Could you check a few things on this drawing? It's one solid part, dimensions in mm from its lowest x, y, z. A direction names the side the tool comes from. Give positions to 0.01 mm unless a question says otherwise; leave off trailing zeros. Order: outer loops, then holes, each group sorted by start corner. A loop starts at its lowest first (then second) coordinate and runs counter-clockwise, first axis right, second up. Notation, with made-up numbers: (-18.5, 29.25) - (39.5, 29.25) arc R37 ccw to (39.5, 66.25) - close; hole circle Ø10 at (89.5, 19.25). An arc over 180 degrees is marked (long way). Return JSON: item names as keys, results as strings.
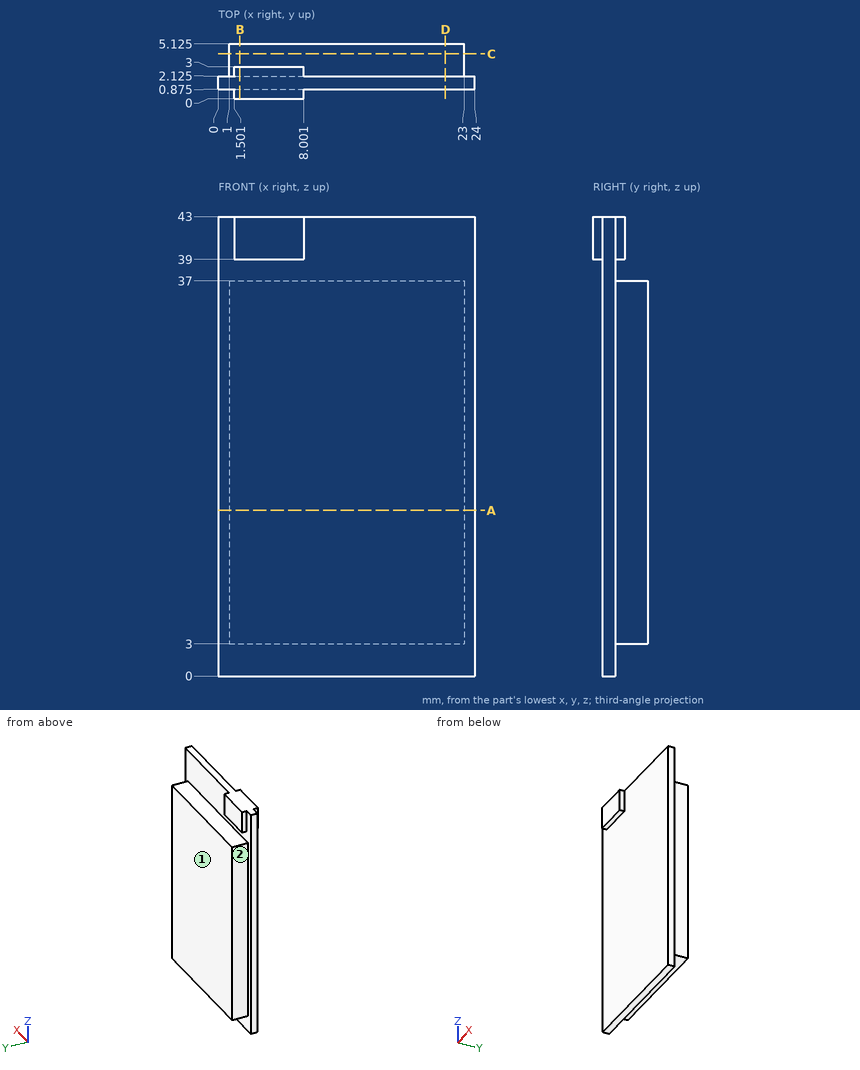
1. Suppose I cut it at A-A (z = 15.5). List the corners of the cut face in (x, y) for me (3 decimals).
Checks:
{"outline": "(0, 0.875) - (24, 0.875) - (24, 2.125) - (23, 2.125) - (23, 5.125) - (1, 5.125) - (1, 2.125) - (0, 2.125) - close"}
2. Suppose I cut it at B-B (x = 2). List the corners of the cut face in (y, z) for me (3 decimals).
Checks:
{"outline": "(0, 39) - (0.875, 39) - (0.875, 0) - (2.125, 0) - (2.125, 3) - (5.125, 3) - (5.125, 37) - (2.125, 37) - (2.125, 39) - (3, 39) - (3, 43) - (0, 43) - close"}
3. If I drill on L1, parallel to Y at x = 10, z = 4.5 (3 decimals); L2, parallel to X at y = 4.85, z = 24.5; L3, parallel to Y at x = 19.5, z = 37.5 (3 decimals), over which ranges is the centre line in solid material (lowest first)? Write a range as [from, to].
Checks:
{"L1": "[0.875, 5.125]", "L2": "[1, 23]", "L3": "[0.875, 2.125]"}
4. Suppose I cut it at D-D (x = 21.25). List the corners of the cut face in (y, z) for me (3 decimals), plus the area to 3 significant figures.
Checks:
{"outline": "(0.875, 0) - (2.125, 0) - (2.125, 3) - (5.125, 3) - (5.125, 37) - (2.125, 37) - (2.125, 43) - (0.875, 43) - close", "area": "156 mm^2"}
5. On a 3-axis mill with a long thin cutter (end or side, diameter ignored), from which of +Z, -Z, +X, -X, +Y, -Y can I reach the whole of each face in a straight line? I mean the marked faces 1 and 2. Say none if no direction works.
Checks:
{"face 1": "+Z, -Z, +X, -X, +Y", "face 2": "+Z, -Z, -X, +Y"}
6. Suppose I cut it at C-C (y = 4.2). List the corners of the cut face in (x, z) for me.
Checks:
{"outline": "(1, 3) - (23, 3) - (23, 37) - (1, 37) - close"}
7. For pin 1 Ø4.5 at (x, z) = (6.5, 40.5) entering from +Y; pin 2 Ø0.9 at (y, z) = (3.5, 26) entering from +X; pin 3 Ø2 at (x, y) = (21, 2) entering from -Z; pin 4 Ø1 at (x, y) = (20, 3.5) entering from +Z, each with a flat end and sliding along its axis, tell me the tip position at first contact or that it passes through.
Checks:
{"pin 1": "y = 3", "pin 2": "x = 23", "pin 3": "z = 0", "pin 4": "z = 37"}
